Part print with two shaded views. Sizes in mm from the minimum x, y, z corner. A direction names the side the tool comes from. Give positions to 0.01 mm unless a question says otherwise; leave off trailing zeros. Write each loop counter-clockwise with the first axis right and the second up, starting at its lowest first coordinate (ties: lowest second). Pieces come first, ordered by that corner, then holes. Notation, with made-up numbers: (67, -17) -> (119, -17) arc R8 cw to (119, -9) -> close; hole circle Ø4 at (2, -11.5). An arc over 180 degrees is marked (long way). Answer as a JSON object with one key per item and string values.
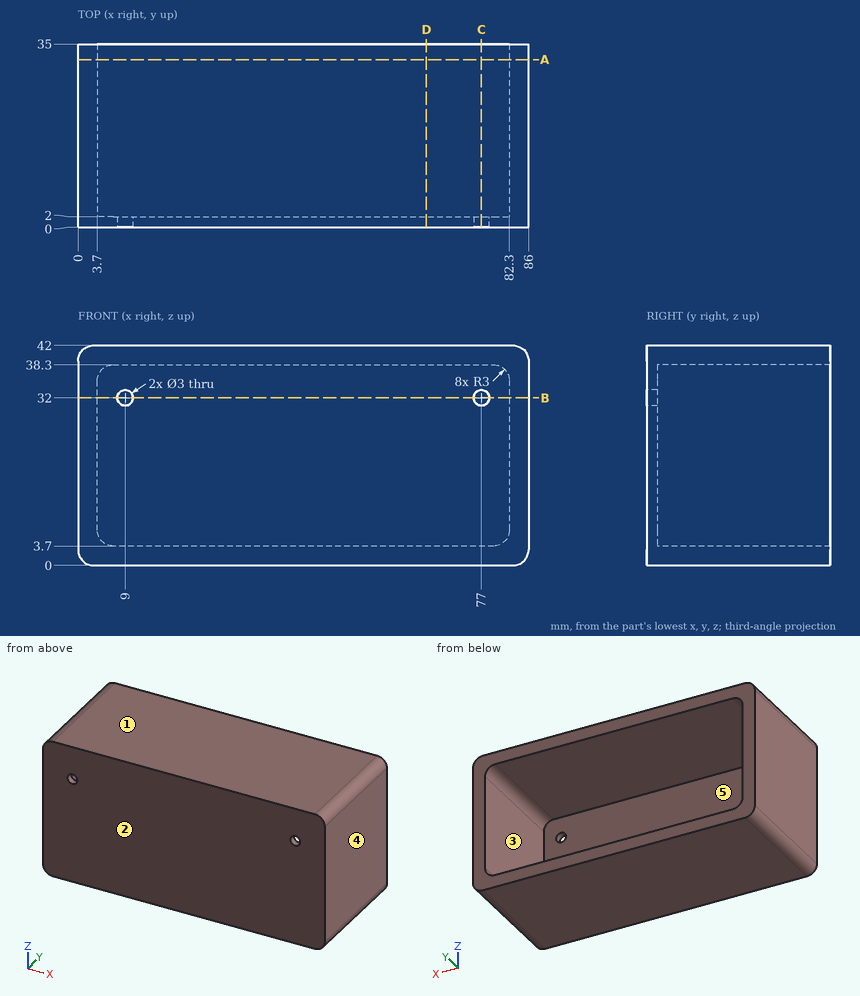
1) Slice it at A-A (y = 32). List the corners of the cut face in (x, z).
Model answer:
{"outline": "(0, 3) arc R3 ccw to (3, 0) -> (83, 0) arc R3 ccw to (86, 3) -> (86, 39) arc R3 ccw to (83, 42) -> (3, 42) arc R3 ccw to (0, 39) -> close; hole (3.7, 6.7) arc R3 ccw to (6.7, 3.7) -> (79.3, 3.7) arc R3 ccw to (82.3, 6.7) -> (82.3, 35.3) arc R3 ccw to (79.3, 38.3) -> (6.7, 38.3) arc R3 ccw to (3.7, 35.3) -> close"}
2) 3-axis set-ups, long thin cutter, end or side, ignore diameter. For the marked faces 4 and 5: which of +Z, -Z, +X, -X, +Y, -Y reach the whole face in a straight line?
Model answer:
{"face 4": "+Z, -Z, +X, +Y, -Y", "face 5": "+Y"}
3) Mould opens along Z. For the marked faces 1, 2 and 3 say: released by +Z, released by -Z, zero draft, split by the parting line, or undercut.
Model answer:
{"face 1": "released by +Z", "face 2": "zero draft", "face 3": "undercut"}
4) Wall check: probe 1 along X at (y, z) = (0.45, 32); probe 2 along Z at (x, y) = (77, 0.9); probe 3 along Z at (x, y) = (6.5, 9). Give the ranges that are in metal, low to high.
Model answer:
{"probe 1": "x = 0 to 7.5, 10.5 to 75.5, 78.5 to 86", "probe 2": "z = 0 to 30.5, 33.5 to 42", "probe 3": "z = 0 to 3.71, 38.29 to 42"}
5) Slice it at C-C (x = 77). List the corners of the cut face in (y, z).
Model answer:
{"outline": "(0, 0) -> (35, 0) -> (35, 3.7) -> (2, 3.7) -> (2, 30.5) -> (0, 30.5) -> close; (0, 33.5) -> (2, 33.5) -> (2, 38.3) -> (35, 38.3) -> (35, 42) -> (0, 42) -> close"}
6) Slice it at B-B (z = 32). List the corners of the cut face in (x, y).
Model answer:
{"outline": "(0, 0) -> (7.5, 0) -> (7.5, 2) -> (3.7, 2) -> (3.7, 35) -> (0, 35) -> close; (10.5, 0) -> (75.5, 0) -> (75.5, 2) -> (10.5, 2) -> close; (78.5, 0) -> (86, 0) -> (86, 35) -> (82.3, 35) -> (82.3, 2) -> (78.5, 2) -> close"}
7) Pin check, flat tips, straight feed: pin 1 (10 mm diameter, centred on x = 76, z = 9, fed in from +Y); pin 2 (2.5 mm diameter, centred on x = 9, z = 32, fed in from +Y). Stop position of each tip, or through.
Model answer:
{"pin 1": "stops at y = 2", "pin 2": "passes through"}
8) Slice it at D-D (x = 66.5). List the corners of the cut face in (y, z).
Model answer:
{"outline": "(0, 0) -> (35, 0) -> (35, 3.7) -> (2, 3.7) -> (2, 38.3) -> (35, 38.3) -> (35, 42) -> (0, 42) -> close"}
